Autodesk Inventor part; units mm, degrees
ref_plane "YZ Plane" through (0, 0, 0) normal (1, 0, 0) x (0, 1, 0)
ref_plane "XZ Plane" through (0, 0, 0) normal (0, 1, 0) x (-1, 0, 0)
ref_plane "XY Plane" through (0, 0, 0) normal (0, 0, 1) x (1, 0, 0)
sketch "Sketch1" plane through (0, 0, 0) normal (0, 1, 0) x (-1, 0, 0)
  line L0 (4.2334, 3.223) -> (-5.7666, 3.223)
  line L1 (-5.7666, 3.223) -> (-5.7666, -6.777)
  line L2 (-5.7666, -6.777) -> (4.2334, -6.777)
  line L3 (4.2334, -6.777) -> (4.2334, 3.223)
  point P0 (0, 0)
  dimension "d0" = 10
  dimension "d1" = 10
extrude "Extrusion1" add sketch "Sketch1" along normal blind 32
sketch "Sketch2" plane through (5.7666, 0, 3.223) normal (1, 0, 0) x (0, 0, -1)
  line L0 (0, 0) -> (10, 0)
  line L1 (0, 0) -> (0, 32)
  line L2 (10, 0) -> (0, 0)
  line L3 (0, 0) -> (0, 10)
  line L4 (0, 10) -> (10, 10)
  line L5 (10, 10) -> (10, 0)
  line L6 (0, 0) -> (-10, 0)
  line L7 (-10, 0) -> (-10, 10)
  line L8 (-10, 10) -> (0, 10)
  line L9 (0, 10) -> (0, 0)
  line L10 (10, 10) -> (20, 10)
  line L11 (20, 10) -> (20, 0)
  line L12 (20, 0) -> (10, 0)
  line L13 (10, 0) -> (10, 10)
  line L14 (-10, 5) -> (0, 10)
  line L15 (10, 10) -> (20, 5)
  point P0 (3.223, 0)
  point P1 (10, 5)
  dimension "d4" = 10
  dimension "d5" = 10
  dimension "d6" = 10
extrude "Extrusion2" add sketch "Sketch2" against normal blind 10 contours L6 L7 L14 L1 | L5 L15 L11 L12
sketch "Sketch3" plane through (5.7666, 32, 3.223) normal (1, 0, 0) x (0, 0, -1)
  line L0 (10, 0) -> (0, 0)
  line L1 (10, -22) -> (10, 0)
  line L2 (0, 0) -> (10, 0)
  line L3 (10, 0) -> (10, -10)
  line L4 (10, -10) -> (0, -10)
  line L5 (0, -10) -> (0, 0)
  line L6 (0, 0) -> (-10, 0)
  line L7 (-10, 0) -> (-10, -10)
  line L8 (-10, -10) -> (0, -10)
  line L9 (0, -10) -> (0, 0)
  line L10 (10, 0) -> (20, 0)
  line L11 (20, 0) -> (20, -10)
  line L12 (20, -10) -> (10, -10)
  line L13 (10, -10) -> (10, 0)
  line L14 (0, -10) -> (-10, -5)
  line L15 (10, -10) -> (20, -5)
  point P0 (3.223, -32)
  point P1 (0, -10)
  dimension "d9" = 10
  dimension "d10" = 10
  dimension "d11" = 10
extrude "Extrusion3" add sketch "Sketch3" against normal blind 10 contours L10 L11 L15 L1 | L5 L14 L7 L6
sketch "Sketch4" plane through (5.7666, 0, -16.777) normal (1, 0, 0) x (0, 0, -1)
  line L0 (-13, 27) -> (-17, 27)
  line L1 (-17, 27) -> (-17, 5)
  line L2 (-17, 5) -> (-13, 5)
  line L3 (-13, 5) -> (-13, 27)
  line L4 (0, 32) -> (-30, 32)
  line L5 (-30, 0) -> (0, 0)
  line L6 (-10, 10) -> (-10, 22)
  line L7 (-20, 10) -> (-20, 22)
  point P0 (-16.777, 0)
  point P1 (-15, 32)
  point P2 (-15, 27)
  point P3 (-15, 5)
  dimension "d14" = 5
  dimension "d15" = 5
  dimension "d16" = 3
  dimension "d17" = 3
extrude "Extrusion4" cut sketch "Sketch4" against normal blind 10
properties part number "stand"
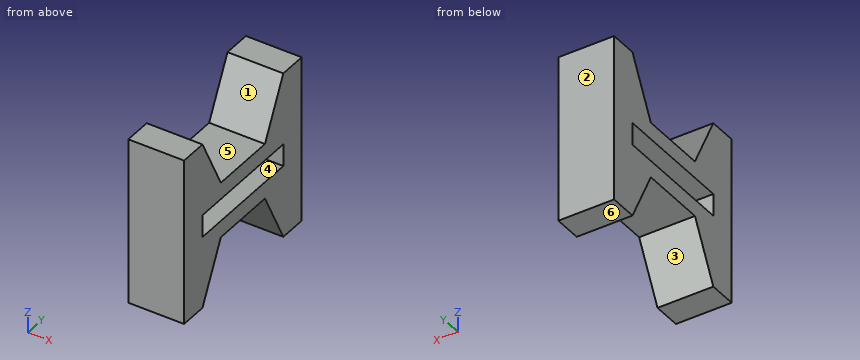
The model under review builds one solid part; all positions refer to its coordinate system, in mm. Face numbers are marked on the shaded views. A direction names the side the tool comes from. Round coordinates to 2 decimals unless told otherwise and drop trailing zeros. Loops run counter-clockwise (first coordinate to the right, second up) from the corner with the lowest first, then second, coordinate; pieces in that order, holes last. Notation, with made-up numbers: (27, 38) - (54, 38) arc R28 cw to (54, 68) - close; hole circle Ø6 at (-9.75, 28). An arc over 180 degrees is marked (long way). Write each question's results on one line, items separated by ' | '. Start each with the question number.
Q1. Draft analysis for pull direction Z (two halves, no side actions). For the marked faces 4, 5 and 6, state which applies: pulls with the +Z half, pulls with the -Z half, needs draft (parallel to the pull), parting line crosses it, or undercut.
Q2. Wall thickness on line 1 along Z through (x, y) = (-0.75, 14); line 2 along Y through (x, z) = (5.25, -0.25); line 3 along Y through (x, z) = (4, -14.25): over which ranges is each line inside the solid? List them lowest first. Write a range as [from, to].
Q3. Take a section at B-B on z = -1.5. Give the boundary of the cut face in (x, y), plus the area to 3 significant figures.
Q4. Tool access review of the marked faces 1, 2 and 3: name each direction out of +Z, -Z, +X, -X, +Y, -Y from which nothing blocks a thin tool from reaching the whole face with its end or side.
Q5. Take a section at C-C on x = 3. Give the boundary of the cut face in (y, z), plus the area to 3 significant figures.
Q6. Insertion check: P1, Ø4.5, axis at x = 2, z = -1, coming from the -Y side; P2, Ø5, axis at x = -3, y = 22.5, coming from the +Z side; P3, Ø3, axis at x = 0.5, y = 15, coming from the -Z side. Each pin has a flat end and moves straight along its axis. Give the tip position at first contact, or say it passes through.
Q7. Take a section at A-A on y = 19. Give the boundary of the cut face in (x, z), plus the area to 3 significant figures.
Data:
1) face 4: undercut | face 5: pulls with the +Z half | face 6: pulls with the -Z half
2) line 1: z = [-6.78, -3.78], [0.22, 3.22] | line 2: y = [0, 5], [27, 32] | line 3: y = [0, 6.26], [25.74, 32]
3) outline: (-4.23, 0) - (5.77, 0) - (5.77, 5) - (-4.23, 5) - close; (-4.23, 27) - (5.77, 27) - (5.77, 32) - (-4.23, 32) - close | area: 100 mm²
4) face 1: +Z, +X, -X | face 2: +Z, -Z, +X, -X, +Y | face 3: -Z, +X, -X
5) outline: (0, -16.78) - (5, -16.78) - (10, -6.78) - (22, -6.78) - (27, -16.78) - (32, -16.78) - (32, 13.22) - (27, 13.22) - (22, 3.22) - (10, 3.22) - (5, 13.22) - (0, 13.22) - close; hole (5, -3.78) - (27, -3.78) - (27, 0.22) - (5, 0.22) - close | area: 532 mm²
6) P1: stops at y = 0 | P2: stops at z = 9.22 | P3: stops at z = -6.78
7) outline: (-4.23, -6.78) - (5.77, -6.78) - (5.77, -3.78) - (-4.23, -3.78) - close; (-4.23, 0.22) - (5.77, 0.22) - (5.77, 3.22) - (-4.23, 3.22) - close | area: 60.0 mm²
